from build123d import *

# Parameters (mm, degrees)
F2_R     = 57.15
F3_DEPTH = 88.9
F0_R     = 57.15
F1_DEPTH = 3.175


# Not quite as in the source:
# - a feature names something its author has since deleted; it is built from what else it names


with BuildPart() as f3:
    # F2 (on Top) → F3 (new body)
    with BuildSketch(Plane.XY):
        with Locations((0, 25.4)):
            Circle(F2_R)
        with BuildLine():
            ThreePointArc((45.7905011984, -3.175), (0, -28.575), (-45.7905011984, -3.175))
            Line((-45.7905011984, -3.175), (45.7905011984, -3.175))
        make_face(mode=Mode.SUBTRACT)
        with BuildLine():
            Line((-22.225, 50.8), (-22.225, 0))
            Line((-22.225, 0), (-28.575, 0))
            ThreePointArc((-28.575, 0), (-53.975, 25.4), (-28.575, 50.8))
            Line((-28.575, 50.8), (-22.225, 50.8))
        make_face(mode=Mode.SUBTRACT)
        Polygon((19.05, 0), (0, 0), (-19.05, 0), (-19.05, 50.8), (0, 50.8), (19.05, 50.8), align=None, mode=Mode.SUBTRACT)
        with BuildLine():
            Line((28.575, 0), (22.225, 0))
            Line((22.225, 0), (22.225, 50.8))
            Line((22.225, 50.8), (28.575, 50.8))
            ThreePointArc((28.575, 50.8), (53.975, 25.4), (28.575, 0))
        make_face(mode=Mode.SUBTRACT)
        with BuildLine():
            Line((45.7905011984, 53.975), (-45.7905011984, 53.975))
            ThreePointArc((-45.7905011984, 53.975), (0, 79.375), (45.7905011984, 53.975))
        make_face(mode=Mode.SUBTRACT)
    extrude(amount=F3_DEPTH)

    # F0 (on face) → F1 (join)
    with BuildSketch(Plane(origin=(0, 0, 0), x_dir=(1, 0, 0), z_dir=(0, 0, -1))):
        with Locations((0, -25.4)):
            Circle(F0_R)
    extrude(amount=F1_DEPTH)


solid = f3.part
CAD build for the part. Positions are in the model's coordinates, mm. A direction names the side the tool comes from. Coordinates: 2 decimals unless noted, no trailing zeros. Write each loop counter-clockwise with the first axis right and the second up, starting at its lowest first coordinate (ties: lowest second). Pieces come first, ordered by that corner, then holes. Notation, with made-up numbers: (-12, -29) - (3, -29) arc R30 cw to (3, -4) - close; hole circle Ø5 at (27.5, -40). An arc over 180 degrees is marked (long way). Use a Markdown table: item, result. Add a question column.
Item 1: Band-saw the part on D-D, the plane y = -17. Give the cut face in (x, z) (3 decimals).
Item 2: 3-axis set-ups, long thin cutter, end or side, ignore diameter. For faces 1 (the face through (25, 0, 44)), 2 (the face through (-1, 25, -3.175)): which of +Z, -Z, +X, -X, +Y, -Y reach the whole face in a straight line?
Item 3: Mould opens along X. For faces 3 (the face through (-21, 30, 88.9)), 4 (the face through (1, 53.975, 44)) say: pulls with the +X half, pulls with the -X half, needs draft (parallel to the pull), parting line crosses it, or undercut.
Item 4: Flat gauge pins, fed straight in: pin 1 (12 mm diameter, centred on y = -17.5, z = 21.5, fed in from -X); pin 2 (1.9 mm diameter, centred on x = 27, z = 64.5, fed in from -Y); pin 3 (3 mm diameter, centred on y = 22, z = 51.5, fed in from +X). Where does each tip first touch, or does it go through?
Item 5: Band-saw the part on A-A, the plane z = 60.5. Give the number of separate pieces and of enclosed holes in the cut face, and give its area (3 significant figures).
Item 6: Drill centre lines: L1, parallel to Y at x = 1, z = 77 (3 decimals); L2, parallel to X at y = 21, z = 1 (3 decimals); L3, parallel to Y at x = 9, z = 78.5 (3 decimals). Where is each one in solid material? Low to high. Write a range as from..to.
Item 7: Band-saw the part on C-C, the plane x = 0. Give the cut face in (y, z) (3 decimals).
Item 8: Band-saw the part on B-B, the plane y = 25.4. Give the cut face in (x, z) (3 decimals), and give its area (3 significant figures).
Numbers:
| question | item | result |
|---|---|---|
| 1 | outline | (-38.319, -3.175) - (38.319, -3.175) - (38.319, 88.9) - (33.4, 88.9) - (33.4, 0) - (-33.4, 0) - (-33.4, 88.9) - (-38.319, 88.9) - close |
| 2 | face 1 | +Z |
| 2 | face 2 | -Z, +X, -X, +Y, -Y |
| 3 | face 3 | needs draft |
| 3 | face 4 | undercut |
| 4 | pin 1 | x = -43.64 |
| 4 | pin 2 | y = -25.47 |
| 4 | pin 3 | x = 57.12 |
| 5 | separate pieces | 1 |
| 5 | enclosed holes | 5 |
| 5 | area | 2,370 mm2 |
| 6 | L1 | -31.741..-28.566, -3.175..0, 50.8..53.975, 79.366..82.541 |
| 6 | L2 | -56.98..-53.591, -22.225..-19.05, 19.05..22.225, 53.591..56.98 |
| 6 | L3 | -31.037..-27.819, -3.175..0, 50.8..53.975, 78.619..81.837 |
| 7 | outline | (-31.75, -3.175) - (82.55, -3.175) - (82.55, 88.9) - (79.375, 88.9) - (79.375, 0) - (53.975, 0) - (53.975, 88.9) - (50.8, 88.9) - (50.8, 0) - (0, 0) - (0, 88.9) - (-3.175, 88.9) - (-3.175, 0) - (-28.575, 0) - (-28.575, 88.9) - (-31.75, 88.9) - close |
| 8 | outline | (-57.15, -3.175) - (57.15, -3.175) - (57.15, 88.9) - (53.975, 88.9) - (53.975, 0) - (22.225, 0) - (22.225, 88.9) - (19.05, 88.9) - (19.05, 0) - (-19.05, 0) - (-19.05, 88.9) - (-22.225, 88.9) - (-22.225, 0) - (-53.975, 0) - (-53.975, 88.9) - (-57.15, 88.9) - close |
| 8 | area | 1,490 mm2 |
